Source: CAD feature listing. Evaluate the final solid. Frame: model axes, mm. Face numbers are marked on the shaded views. A direction names the side the tool comes from. Give positions to 0.01 mm unless a question says otherwise; leave off trailing zeros. Order: outer loops, then holes, each group sorted by start corner. A loop starts at its lowest first (then second) coordinate and runs counter-clockwise, first axis right, second up. Notation, with made-up numbers: M 50,-36 L 99,-36 A5 ccw 99,-29 Z; hole C 26,63.25 d7. An arc over 180 degrees is marked long. Answer in a Markdown table with one row per item. Add a question column.
(1) Pin query (flat end, axial travel): P1, Ø8, axis at x = -315.5, z = 81, coming from the -Y side; P2, Ø8, axis at x = 2.5, y = -331, coming from the +Z side. Return the tip coordinate at first contact, or that it passes through.
(2) Section query D-D, the plane y = -303.5. Return loops of the section in (x, z).
(3) Material intervals for line 1 along X through (y, z) = (-111, 129); line 2 along Y through (x, z) = (156.5, -106); line 3 along X through (y, z) = (-547.5, -297.5), sorted ascending.
(4) Section query A-A, the plane z = 149. Return loops of the section in (x, y).
(5) Mould query, pull axis X, two halves, no side actions, for the marked faces 4, 5 and 6. Classes: pulls with the +X half, pulls with the -X half, needs draft (parallel to the pull), parting line crosses it, or undercut.
(6) Section query B-B, the plane y = -512. Return loops of the section in (x, z), plus the area to 3 significant figures.
(7) Section query C-C, the plane x = 313.5. Return loops of the section in (y, z).
(8) Set-up query: the marked faces 1, 2 and 3. Return all of +Z, -Z, +X, -X, +Y, -Y with unobstructed straight access to the full face (end or side cutting, diameter ignored); none if empty.
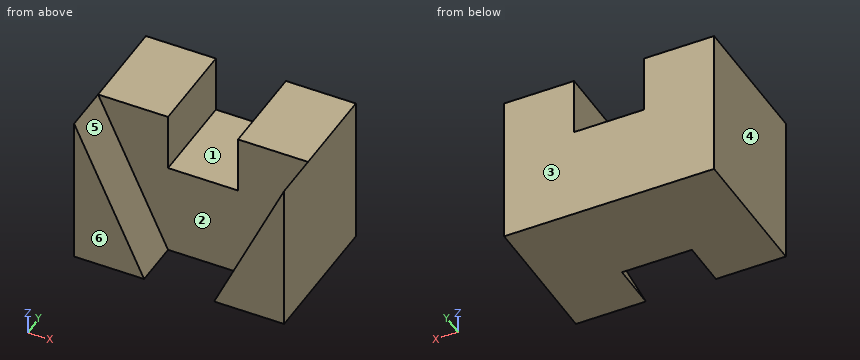
from build123d import *

# Parameters (mm, degrees)
F0_W     = 900
F0_H     = 650
F1_DEPTH = 400
F2_W     = 300
F2_H     = 250
F3_DEPTH = 400.001
F5_DEPTH = 200


with BuildPart() as f1:
    # F0 (on Front) → F1 (new body)
    with BuildSketch(Plane.XZ):
        Rectangle(F0_W, F0_H)
    extrude(amount=F1_DEPTH)

    # F2 (on face) → F3 (cut, through all)
    with BuildSketch(Plane.XZ.offset(400)):
        with Locations((0, 200)):
            Rectangle(F2_W, F2_H)
    extrude(amount=-F3_DEPTH, mode=Mode.SUBTRACT)

    # F4 (on face) → F5 (join)
    with BuildSketch(Plane.XZ.offset(400)):
        Polygon((-150, -325), (-450, 325), (-450, -325), align=None)
        Polygon((450, -325), (450, 325), (150, -325), align=None)
    extrude(amount=F5_DEPTH)


solid = f1.part
Values follow:
| question | item | result |
|---|---|---|
| 1 | P1 | stops at y = -400 |
| 1 | P2 | stops at z = 75 |
| 2 | outline | M -450,-325 L 450,-325 L 450,325 L 150,325 L 150,75 L -150,75 L -150,325 L -450,325 Z |
| 3 | line 1 | x = -450 to -150, 150 to 450 |
| 3 | line 2 | y = -400 to 0 |
| 3 | line 3 | x = -450 to -162.69, 162.69 to 450 |
| 4 | outline | M -450,-600 L -368.77,-600 L -368.77,-400 L -150,-400 L -150,0 L -450,0 Z; M 150,-400 L 368.77,-400 L 368.77,-600 L 450,-600 L 450,0 L 150,0 Z |
| 5 | face 4 | pulls with the -X half |
| 5 | face 5 | undercut |
| 5 | face 6 | needs draft |
| 6 | outline | M -450,-325 L -150,-325 L -450,325 Z; M 150,-325 L 450,-325 L 450,325 Z |
| 6 | area | 195,000 mm² |
| 7 | outline | M -600,-325 L 0,-325 L 0,325 L -400,325 L -400,29.25 L -600,29.25 Z |
| 8 | face 1 | +Z, +Y, -Y |
| 8 | face 2 | +Z, -Y |
| 8 | face 3 | +Z, -Z, +X, -X, +Y |
